from build123d import *

# Parameters (mm, degrees)
SKETCH_1_R           = 15
SKETCH_1_R_2         = 10
EXTRUDE_1_DEPTH      = 7.5
EXTRUDE_2_REACH      = 64.3
EXTRUDE_2_END_RADIUS = 15
SKETCH_3_R           = 5
SKETCH_4_W           = 30
SKETCH_4_H           = 30
EXTRUDE_3_DEPTH      = 15
SKETCH_5_R           = 2
CUT_EXTRUDE_1_DEPTH  = 78.942286456


with BuildPart() as part:
    # 草图1 → 凸台-拉伸1 (new, symmetric)
    with BuildSketch(Plane.XY):
        Circle(SKETCH_1_R)
        Circle(SKETCH_1_R_2, mode=Mode.SUBTRACT)
    extrude(amount=EXTRUDE_1_DEPTH, both=True)

    # 凸台-拉伸2: up to this cylinder (the profile starts outside it)
    extrude_2_end = Plane(origin=(0, 0, 0), z_dir=(0, 0, -1)) * Cylinder(EXTRUDE_2_END_RADIUS, 159.6, mode=Mode.PRIVATE)
    # 草图3 → 凸台-拉伸2 (add, up to the surface)
    with BuildSketch(Plane(origin=(0, 45, 0), x_dir=(1, 0, 0), z_dir=(0, 1, 0)), mode=Mode.PRIVATE) as extrude_2_sk1:
        with Locations(Location((0, 0, 0), (0, 0, 270))):
            Circle(SKETCH_3_R)
    extrude_2_tool1 = extrude(extrude_2_sk1.sketch, amount=-EXTRUDE_2_REACH, mode=Mode.PRIVATE) - extrude_2_end
    add(extrude_2_tool1.solids().sort_by_distance((0, 45, 0))[0])

    # 草图4 → 凸台-拉伸3 (add)
    with BuildSketch(Plane(origin=(0, 45, 0), x_dir=(1, 0, 0), z_dir=(0, 1, 0))):
        Rectangle(SKETCH_4_W, SKETCH_4_H)
    extrude(amount=EXTRUDE_3_DEPTH)

    # 草图5 → 切除-拉伸1 (cut, through all)
    with BuildSketch(Plane(origin=(0, 60, 0), x_dir=(1, 0, 0), z_dir=(0, 1, 0))):
        with Locations(Location((10, 10, 0), (0, 0, 270))):
            Circle(SKETCH_5_R)
        with Locations(Location((-10, 10, 0), (0, 0, 270))):
            Circle(SKETCH_5_R)
        with Locations(Location((10, -10, 0), (0, 0, 270))):
            Circle(SKETCH_5_R)
        with Locations(Location((-10, -10, 0), (0, 0, 270))):
            Circle(SKETCH_5_R)
    extrude(amount=-CUT_EXTRUDE_1_DEPTH, mode=Mode.SUBTRACT)


solid = part.part
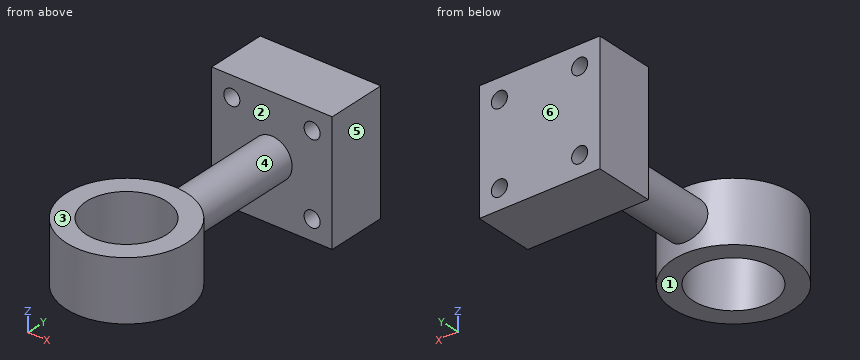
Verification items for the finished model (mm, model axes). Face numbers are marked on the shaded views. A direction names the side the tool comes from. Coordinates: 2 decimals unless noted, no trailing zeros. Order: outer loops, then holes, each group sorted by start corner. A loop starts at its lowest first (then second) coordinate and runs counter-clockwise, first axis right, second up.
Item 1: Section check D-D, the plane y = -6. Enter the section's corners in (x, z), then the cut area to 3 significant figures.
Filled in:
outline: (-13.75, -7.5) - (-8, -7.5) - (-8, 7.5) - (-13.75, 7.5) - close; (8, -7.5) - (13.75, -7.5) - (13.75, 7.5) - (8, 7.5) - close
area: 172 mm2
Item 2: Access from +Z, -Z, +X, -X, +Y, -Y to the whole of each face (thin tool, end or side, straight path). Record for the marked faces 1, 2 and 3.
Filled in:
face 1: -Z, +X, -X, -Y
face 2: none
face 3: +Z, +X, -X, -Y
Item 3: Section check A-A, the plane z = 10. Enter the section's corners in (x, y), then the cut area to 3 significant figures.
Filled in:
outline: (-15, 45) - (-12, 45) - (-12, 60) - (-15, 60) - close; (-8, 45) - (8, 45) - (8, 60) - (-8, 60) - close; (12, 45) - (15, 45) - (15, 60) - (12, 60) - close
area: 330 mm2
Item 4: Section check B-B, the plane x = 0. Enter the section's corners in (y, z).
Filled in:
outline: (-15, -7.5) - (-10, -7.5) - (-10, 7.5) - (-15, 7.5) - close; (10, -7.5) - (15, -7.5) - (15, -5) - (45, -5) - (45, -15) - (60, -15) - (60, 15) - (45, 15) - (45, 5) - (15, 5) - (15, 7.5) - (10, 7.5) - close
Item 5: Depth check by flat-ended pin: pin 1 (1.5 mm diameter, centred on y = 32, z = -1.5, fed in from -X); pin 2 (12 mm diameter, centred on x = 0, y = 0, fed in from -Z); pin 3 (1 mm diameter, centred on x = 9.5, z = 0.5, fed in from -Y); pin 4 (9 mm diameter, centred on x = -6.5, y = 2, fed in from +Z). Enter the tip coordinate at first touch or a pass-through.
Filled in:
pin 1: stops at x = -4.94
pin 2: passes through
pin 3: stops at y = -12
pin 4: stops at z = 7.5
Item 6: Release check for a two-part mould opening along Y. For the marked faces 4, 5 and 6 record: +Y half, -Y half, draft (parallel to the pull), parting line (faces both ways), or undercut.
Filled in:
face 4: undercut
face 5: draft
face 6: +Y half
Item 7: Material ranges on L1, parallel to X at y = 48, z = -10; L2, parallel to Y at x = -3, z = 4.25; L3, parallel to Y at x = -7.5, z = 6, recorded low to high.
Filled in:
L1: x = -15 to -12, -8 to 8, 12 to 15
L2: y = -14.7 to -9.54, 9.54 to 14.7, 45 to 60
L3: y = -12.99 to -6.61, 6.61 to 12.99, 45 to 60
Item 8: Section check C-C, the plane z = 6.75. Enter the section's corners in (x, y), then the cut area to 3 significant figures.
Filled in:
outline: circle Ø30 at (0, 0); (-15, 45) - (15, 45) - (15, 60) - (-15, 60) - close; hole circle Ø20 at (0, 0)
area: 843 mm2
